The model under review builds one solid part; all positions refer to its coordinate system, in mm. A direction names the side the tool comes from. Coordinates: 2 decimals unless noted, no trailing zeros. Use CSV: the item, a comma, the result in double quotes. Start each with the question number.
1. Clearance check with flat-ended pins moving along their axes: P1, Ø1.5, axis at x = -3.5, z = -16, coming from the -Y side; P2, Ø3, axis at y = 12, z = -29, coming from the -X side; P3, Ø12, axis at x = -16.5, y = 10, coming from the +Z side; P4, Ø6, axis at y = 3, z = -24, coming from the -X side. State where each tip first meets the part, or that it passes through.
2. Draft analysis for pull direction Z (two halves, no side actions). For faces 4 (the flat face through (-17.3, 0, -0.6)), 5 (the flat face through (-15.787, 2.636, -30.966)), 6 (the flat face through (-16.09, 14.33, -4.69)), state which applies: +Z half, -Z half, draft (parallel to the pull), parting line (faces both ways), or undercut.
3. For L1, parallel to Y at x = -19, z = -16.5; L2, parallel to Y at x = -30, z = -19; L3, parallel to X at y = 10.25, z = -5.5, list the stretches that pass through material, from the lowest coordinate up.
4. Tool access review of faces 1 (the flat face through (-16.213, 2.636, -1.034)), 2 (the flat face through (-16, 24, -16)), 3 (the flat face through (-16, 6, -2)): name each direction out of +Z, -Z, +X, -X, +Y, -Y from which nothing blocks a thin tool from reaching the whole face with its end or side.
from build123d import *

# Parameters (mm, degrees)
SKETCH1_W           = 32
SKETCH1_H           = 32
BOSS_EXTRUDE1_DEPTH = 6
BOSS_EXTRUDE1_TAPER = 5
SKETCH2_W           = 26
SKETCH2_H           = 26
BOSS_EXTRUDE2_DEPTH = 18
BOSS_EXTRUDE2_TAPER = 5
SHELL1_T            = -0.8


with BuildPart() as part:
    # Sketch1 → Boss-Extrude1 (new body)
    with BuildSketch(Plane(origin=(0, 0, 0), x_dir=(1, 0, 0), z_dir=(0, 1, 0))):
        with Locations((-16, 16)):
            Rectangle(SKETCH1_W, SKETCH1_H)
    extrude(amount=BOSS_EXTRUDE1_DEPTH, taper=BOSS_EXTRUDE1_TAPER)

    # Sketch2 → Boss-Extrude2 (add)
    with BuildSketch(Plane(origin=(0, 6, 0), x_dir=(1, 0, 0), z_dir=(0, 1, 0))):
        with Locations((-15.92307672, 16.156742102)):
            Rectangle(SKETCH2_W, SKETCH2_H)
    extrude(amount=BOSS_EXTRUDE2_DEPTH, taper=BOSS_EXTRUDE2_TAPER)

    # Shell1
    shell1_openings = [part.faces().sort_by_distance(p)[0] for p in [
        (-16, 0, -16),
    ]]
    offset(amount=SHELL1_T, openings=shell1_openings, kind=Kind.INTERSECTION)


solid = part.part
Computed:
1,P1,"stops at y = 5.2"
1,P2,"stops at x = -28.53"
1,P3,"stops at z = -0.35"
1,P4,"stops at x = -32"
2,face 4,"draft"
2,face 5,"undercut"
2,face 6,"undercut"
3,L1,"y = 23.2 to 24"
3,L2,"y = 5.2 to 6"
3,L3,"x = -28.55 to -27.75, -4.1 to -3.29"
4,face 1,"-Y"
4,face 2,"+Z, -Z, +X, -X, +Y"
4,face 3,"+Y"
